Build history of the part. All positions in model axes, mm. Face numbers are marked on the shaded views. A direction names the side the tool comes from. Give positions to 0.01 mm unless a question says otherwise; leave off trailing zeros. Order: outer loops, then holes, each group sorted by start corner. A loop starts at its lowest first (then second) coordinate and runs counter-clockwise, first axis right, second up. Notation, with made-up numbers: (-3.75, -18) - (23.25, -18) arc R29 ccw to (23.25, 20) - close; hole circle Ø10 at (0.25, -37). An arc over 180 degrees is marked (long way). Use a Markdown table: item, result. Add a question column.
(1) Slice it at D-D (z = 17.5). Write the cut outline in (x, y).
(2) Slice it at A-A (y = -11.5). Write the cut outline in (x, z), then the cut area to 3 significant figures.
(3) Which spindle directions (+Z, -Z, +X, -X, +Y, -Y) get a long thin tool onto all of the face, cutting with end or side? Do the marked faces 1 and 2. Say none if no direction does.
(4) Slice it at C-C (x = 47). Write the cut outline in (y, z) (3 decimals), then the cut area to 3 significant figures.
(5) Flat gauge pins, fed straight in: pin 1 (3 mm diameter, centred on x = 60, y = 10, fed in from +Z); pin 2 (8 mm diameter, centred on x = 25, z = -16, fed in from -Y); pin 3 (2 mm diameter, centred on x = 32.5, y = -8, fed in from -Z). Where does each tip first touch, or does it go through?
(6) Slice it at B-B (z = 0). Write the cut outline in (x, y) (3 decimals), then the cut area to 3 significant figures.
(7) Mould opens along Y. For the marked faces 3, 4 and 5 say: +Y half, -Y half, draft (parallel to the pull), parting line (faces both ways), or undercut.
(8) Wall check: line 1 (Z direction, x = 47.5, y = 0) (3 decimals); line 2 (Z direction, x = 43, y = 12.5); line 3 (Y direction, x = 13.5, z = 6). Give the ranges that are in metal, low to high.
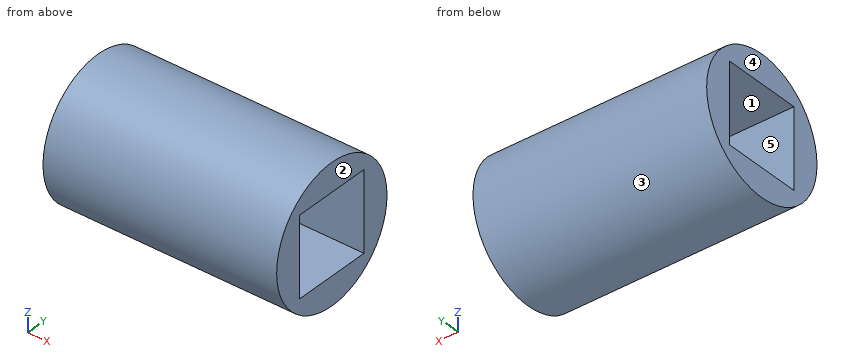
Autodesk Inventor part; units mm, degrees
ref_plane "YZ Plane" through (0, 0, 0) normal (1, 0, 0) x (0, 1, 0)
ref_plane "XZ Plane" through (0, 0, 0) normal (0, 1, 0) x (-1, 0, 0)
ref_plane "XY Plane" through (0, 0, 0) normal (0, 0, 1) x (1, 0, 0)
sketch "Sketch1" plane through (0, 0, 0) normal (1, 0, 0) x (0, 1, 0)
  circle A0 centre (0, 0) radius 22.225
  line L0 (12.954, 12.954) -> (-12.954, 12.954)
  line L1 (-12.954, 12.954) -> (-12.954, -12.954)
  line L2 (-12.954, -12.954) -> (12.954, -12.954)
  line L3 (12.954, -12.954) -> (12.954, 12.954)
  dimension "d0" = 44.45
  dimension "d1" = 25.908
  dimension "d2" = 25.908
extrude "Extrusion1" add sketch "Sketch1" along normal blind 76.2
properties part number "220411 Small Rod Plain"
Solution:
| question | item | result |
|---|---|---|
| 1 | outline | (0, -13.7) - (76.2, -13.7) - (76.2, 13.7) - (0, 13.7) - close |
| 2 | outline | (0, -19.02) - (76.2, -19.02) - (76.2, -12.95) - (0, -12.95) - close; (0, 12.95) - (76.2, 12.95) - (76.2, 19.02) - (0, 19.02) - close |
| 2 | area | 924 mm2 |
| 3 | face 1 | +X, -X |
| 3 | face 2 | +Z, -Z, +X, +Y, -Y |
| 4 | outline | circle Ø44.45 at (0, 0); hole (-12.954, -12.954) - (12.954, -12.954) - (12.954, 12.954) - (-12.954, 12.954) - close |
| 4 | area | 881 mm2 |
| 5 | pin 1 | z = 20.54 |
| 5 | pin 2 | y = -18.71 |
| 5 | pin 3 | z = -21.09 |
| 6 | outline | (0, -22.225) - (76.2, -22.225) - (76.2, -12.954) - (0, -12.954) - close; (0, 12.954) - (76.2, 12.954) - (76.2, 22.225) - (0, 22.225) - close |
| 6 | area | 1,410 mm2 |
| 7 | face 3 | parting line |
| 7 | face 4 | draft |
| 7 | face 5 | undercut |
| 8 | line 1 | -22.225 to -12.954, 12.954 to 22.225 |
| 8 | line 2 | -18.38 to -12.95, 12.95 to 18.38 |
| 8 | line 3 | -21.4 to -12.95, 12.95 to 21.4 |
